```python
from build123d import *

# Parameters (mm, degrees)
F2_R = 2


with BuildPart() as f1:
    # F0 (on Front) → F1 (revolve)
    with BuildSketch(Plane.XZ):
        Polygon((-4, 0), (0, 0), (0, 36.851066), (-4, 36.851066), (-4, 30), (-10, 30), (-10, 5), (-4, 5), align=None)
    revolve(axis=Axis((0, 0, 18.425533), (0, 0, -1)))

    # F2
    f2_edges = [f1.edges().sort_by_distance(p)[0] for p in [
        (10, 0, 30),
        (10, 0, 5),
        (4, 0, 0),
        (4, 0, 36.851066),
    ]]
    fillet(f2_edges, radius=F2_R)


solid = f1.part
```
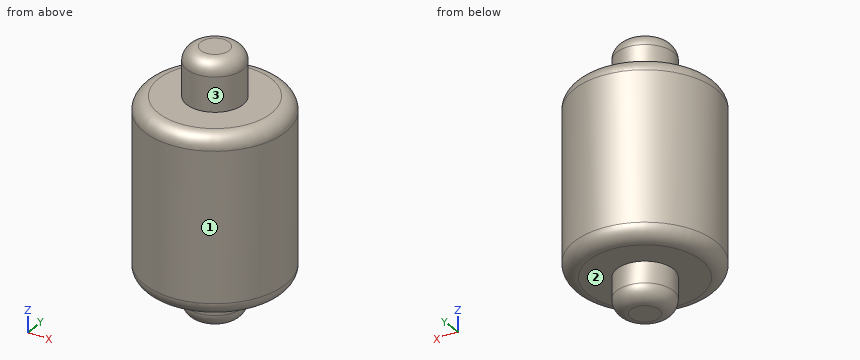
Part model, mm, in its own coordinate system. Face numbers are marked on the shaded views. A direction names the side the tool comes from. Coordinates: 2 decimals unless noted, no trailing zeros. Order: outer loops, then holes, each group sorted by start corner. A loop starts at its lowest first (then second) coordinate and runs counter-clockwise, first axis right, second up. Notation, with made-up numbers: (50, 68) -> (59, 68) arc R23 ccw to (59, 95) -> close; hole circle Ø10 at (38.25, 52). An arc over 180 degrees is marked (long way). Put each result on its own line as item: value. Start each with the question number.
(1) Band-saw the part on A-A (z = 17). Give the cut face in (x, y).
(2) Probe line 1 along Z through (x, y) = (-8, 0); line 2 along Y through (x, z) = (-6, 8.5); line 3 along Y through (x, z) = (-8.75, 27). List the from-to ranges inside material, lowest first. Write a range as [from, to].
(3) Which spindle directions (+Z, -Z, +X, -X, +Y, -Y) get a long thin tool onto all of the face, cutting with end or side? Do the marked faces 1, 2 and 3. Say none if no direction does.
(4) Pin check, flat tips, straight feed: pin 1 Ø3 at (y, z) = (1, 30) entering from +X; pin 2 Ø2 at (x, y) = (3, -6.5) entering from -Z; pin 3 Ø1 at (x, z) = (6.5, 7.5) entering from +Y. Stop position of each tip, or through.
Determined:
1. outline: circle Ø20 at (0, 0)
2. line 1: z = [5, 30]
2. line 2: y = [-8, 8]
2. line 3: y = [-4.84, 4.84]
3. face 1: +Z, -Z
3. face 2: -Z
3. face 3: +Z
4. pin 1: stops at x = 9.9
4. pin 2: stops at z = 5
4. pin 3: stops at y = 8
